Could you check a few things on this model? Use its own coordinates, in mm. A direction names the side the tool comes from. Round coordinates to 2 decimals unless told otherwise and drop trailing zeros. Write each loop counter-clockwise with the first axis right and the second up, starting at its lowest first coordinate (ties: lowest second). Pieces come first, ordered by that corner, then holes.
```python
from build123d import *

# Parameters (mm, degrees)
F0_W     = 82
F0_H     = 41
F1_DEPTH = 2
F0_W_2   = 86
F0_H_2   = 45
F2_DEPTH = 25
F3_R     = 5
F4_D     = 5


with BuildPart() as f1:
    # F0 (on Front) → F1 (new body)
    with BuildSketch(Plane.XZ):
        Rectangle(F0_W, F0_H)
    extrude(amount=F1_DEPTH)

    # F0 (on Front) → F2 (join)
    with BuildSketch(Plane.XZ):
        Rectangle(F0_W_2, F0_H_2)
        Rectangle(F0_W, F0_H, mode=Mode.SUBTRACT)
    extrude(amount=F2_DEPTH)

    # F3
    f3_edges = [f1.edges().sort_by_distance(p)[0] for p in [
        (43, -12.5, 22.5),
        (-43, -12.5, -22.5),
        (-43, -12.5, 22.5),
        (43, -12.5, -22.5),
        (41, -13.5, -20.5),
        (-41, -13.5, -20.5),
        (41, -13.5, 20.5),
        (-41, -13.5, 20.5),
    ]]
    fillet(f3_edges, radius=F3_R)

    # F4 (through all)
    with Locations(Plane(origin=(0, 0, 0), x_dir=(1, 0, 0), z_dir=(0, 1, 0))):
        with Locations((0, 0)):
            Hole(F4_D / 2)


solid = f1.part
```
Q1. If I drill on L1, parallel to Z at x = 30.5, y = -10.75; L2, parallel to Z at x = 0, y = -1.3; L3, parallel to X at y = -2.25, z = -12, over which ranges is the centre line in solid material (lowest first)?
Q2. On a 3-axis mill with a long thin cutter (end or side, diameter ignored), from which of +Z, -Z, +X, -X, +Y, -Y can I reach the whole of each face in a straight line? I mean faces 1 (the flat face through (0, -25, 22)), 2 (the cylindrical face through (39.5, -13.66, -19.07)). Say none if no direction works.
Q3. Imagine slicing it at B-B, the plane x = 0. Write out the boundary of the cut face in (y, z), then the cut area to 3 significant figures.
Q4. Imagine slicing it at D-D, the plane z = -11.5. Write out the boundary of the cut face in (x, y).
Q5. I'm going to push flat-ended pins straight in: pin 1 Ø1.5 at (x, z) = (-16, -18) entering from +Y; pin 2 Ø2 at (x, z) = (1.5, -12) entering from -Y. Where does each tip first touch, or does it pass through?
Q6. Imagine slicing it at C-C, the plane y = -16.25. Write out the boundary of the cut face in (x, z), then the cut area to 3 significant figures.
Q7. We'd pull the mould along Z, two halves only. Please class faces 3 (the flat face through (43, -12, 0)), 4 (the cylindrical face through (-41.57, -12.68, -21)), 5 (the flat face through (-41, -13, 0)): pulls with the +Z half, pulls with the -Z half, needs draft (parallel to the pull), parting line crosses it, or undercut.
Q8. Imagine slicing it at A-A, the plane z = 0. Write out the boundary of the cut face in (x, y), then the cut area to 3 significant figures.
Results found:
1. L1: z = -22.5 to -20.5, 20.5 to 22.5
1. L2: z = -22.5 to -2.5, 2.5 to 22.5
1. L3: x = -43 to -41, 41 to 43
2. face 1: +Z, -Z, +X, -X, -Y
2. face 2: -Y
3. outline: (-25, -22.5) - (0, -22.5) - (0, -2.5) - (-2, -2.5) - (-2, -20.5) - (-25, -20.5) - close; (-25, 20.5) - (-2, 20.5) - (-2, 2.5) - (0, 2.5) - (0, 22.5) - (-25, 22.5) - close
3. area: 172 mm2
4. outline: (-43, -25) - (-41, -25) - (-41, -2) - (41, -2) - (41, -25) - (43, -25) - (43, 0) - (-43, 0) - close
5. pin 1: stops at y = 0
5. pin 2: stops at y = -2
6. outline: (-43, -17.5) arc R5 ccw to (-38, -22.5) - (38, -22.5) arc R5 ccw to (43, -17.5) - (43, 17.5) arc R5 ccw to (38, 22.5) - (-38, 22.5) arc R5 ccw to (-43, 17.5) - close; hole (-41, -15.5) arc R5 ccw to (-36, -20.5) - (36, -20.5) arc R5 ccw to (41, -15.5) - (41, 15.5) arc R5 ccw to (36, 20.5) - (-36, 20.5) arc R5 ccw to (-41, 15.5) - close
6. area: 508 mm2
7. face 3: needs draft
7. face 4: pulls with the -Z half
7. face 5: undercut
8. outline: (-43, -25) - (-41, -25) - (-41, -2) - (-2.5, -2) - (-2.5, 0) - (-43, 0) - close; (2.5, -2) - (41, -2) - (41, -25) - (43, -25) - (43, 0) - (2.5, 0) - close
8. area: 254 mm2
